from build123d import *


with BuildPart() as part:
    # Sketch1 → Base-Revolve (revolve)
    with BuildSketch(Plane.XY):
        with BuildLine():
            Line((0, 12.25), (0, 16.5))
            ThreePointArc((0, 16.5), (-0.146446609, 16.853553391), (-0.5, 17))
            Line((-0.5, 17), (-12.5, 17))
            ThreePointArc((-12.5, 17), (-12.853553391, 17.146446609), (-13, 17.5))
            Line((-13, 17.5), (-13, 19.5))
            ThreePointArc((-13, 19.5), (-13.146446609, 19.853553391), (-13.5, 20))
            Line((-13.5, 20), (-19, 20))
            ThreePointArc((-19, 20), (-20.414213562, 19.414213562), (-21, 18))
            Line((-21, 18), (-21, 12.25))
            Line((-21, 12.25), (-19.6675, 10.9175))
            Line((-19.6675, 10.9175), (-1.3325, 10.9175))
            Line((-1.3325, 10.9175), (0, 12.25))
        make_face()
    revolve(axis=Axis((0, 0, 0), (-1, 0, 0)))


solid = part.part
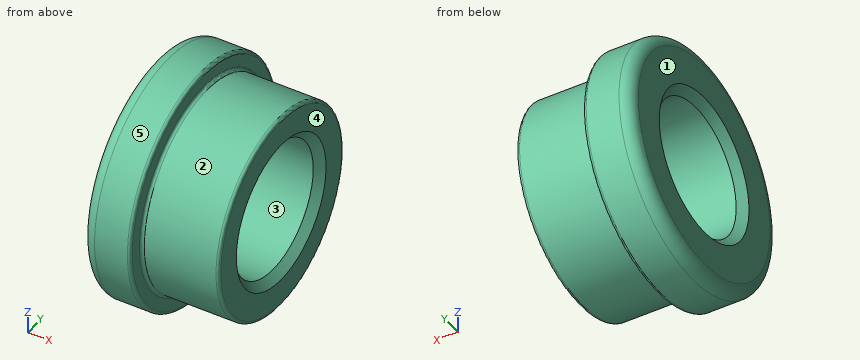
Geometry check sheet. Reference: the model listing, model coordinates, mm. Face numbers are marked on the shaded views. A direction names the side the tool comes from. Give positions to 0.01 mm unless a question says otherwise; leave off trailing zeros. Order: outer loops, then holes, each group sorted by start corner. A loop starts at its lowest first (then second) coordinate and runs counter-clockwise, first axis right, second up.
1. Sectioned sample at C-C (x = -8.5). Record the boundary of the cut face in (y, z) (1 decimal), then the cut area to 3 significant figures.
Completed:
outline: circle Ø34 at (0, 0); hole circle Ø21.8 at (0, 0)
area: 533 mm2
2. Access from +Z, -Z, +X, -X, +Y, -Y to the whole of each face (thin tool, end or side, straight path). Record for the marked faces 1 and 2.
Completed:
face 1: +Z, -Z, -X, +Y, -Y
face 2: +X
3. Draft check along Z on the marked faces 3, 4 and 5. Enter one of: pulls with the +Z half, pulls with the -Z half, needs draft (parallel to the pull), parting line crosses it, or undercut.
Completed:
face 3: undercut
face 4: needs draft
face 5: parting line crosses it
4. Scan lines: line 1 (Y direction, x = -11, z = 0); line 2 (Z direction, x = -13.5, y = 0). Record each from-to range of solid material in increasing order.
Completed:
line 1: y = -17 to -10.92, 10.92 to 17
line 2: z = -20 to -10.92, 10.92 to 20
5. Depth check by flat-ended pin: pin 1 (6 mm diameter, centred on x = -5, z = -11.5, fed in from +Y); pin 2 (8 mm diameter, centred on x = -16.5, z = -6.5, fed in from -Y); pin 3 (2 mm diameter, centred on y = -13.5, z = -11.5, fed in from +X). Enter the tip coordinate at first touch or a pass-through.
Completed:
pin 1: stops at y = 14.72
pin 2: stops at y = -19.84
pin 3: stops at x = -0.06
6. Sectioned sample at A-A (z = 0). Record the boundary of the cut face in (x, y).
Completed:
outline: (-21, -18) arc R2 ccw to (-19, -20) - (-13.5, -20) arc R0.5 ccw to (-13, -19.5) - (-13, -17.5) arc R0.5 cw to (-12.5, -17) - (-0.5, -17) arc R0.5 ccw to (0, -16.5) - (0, -12.25) - (-1.33, -10.92) - (-19.67, -10.92) - (-21, -12.25) - close; (-21, 12.25) - (-19.67, 10.92) - (-1.33, 10.92) - (0, 12.25) - (0, 16.5) arc R0.5 ccw to (-0.5, 17) - (-12.5, 17) arc R0.5 cw to (-13, 17.5) - (-13, 19.5) arc R0.5 ccw to (-13.5, 20) - (-19, 20) arc R2 ccw to (-21, 18) - close
